```python
from build123d import *

# Parameters (mm, degrees)
SKETCH1_R               = 2.75
SKETCH1_R_2             = 1.5
BOSS_EXTRUDE1_DEPTH     = 4.5
SKETCH2_R               = 2.75
BOSS_EXTRUDE2_DEPTH     = 1
SKETCH4_R               = 3.75
BOSS_EXTRUDE3_DEPTH     = 6
CUT_EXTRUDE2_DEPTH      = 14.578475761
CUT_EXTRUDE2_DEPTH_BACK = 14.578475761
CUT_EXTRUDE3_DEPTH      = 14.336978811
CUT_EXTRUDE3_DEPTH_BACK = 14.336978811
CUT_EXTRUDE4_DEPTH      = 14.336978811
CUT_EXTRUDE4_DEPTH_BACK = 14.336978811
SKETCH7_R               = 1.5
SKETCH9_R               = 1.5
CUT_EXTRUDE5_DEPTH      = 14.336978811


with BuildPart() as part:
    # Sketch1 → Boss-Extrude1 (new body)
    with BuildSketch(Plane(origin=(0, 0, 0), x_dir=(1, 0, 0), z_dir=(0, 1, 0))):
        with Locations(Location((0, 0, 0), (0, 0, 270))):
            Circle(SKETCH1_R)
        with Locations(Location((0, 0, 0), (0, 0, 270))):
            Circle(SKETCH1_R_2, mode=Mode.SUBTRACT)
    extrude(amount=BOSS_EXTRUDE1_DEPTH)

    # Sketch2 → Boss-Extrude2 (add)
    with BuildSketch(Plane(origin=(0, 4.5, 0), x_dir=(1, 0, 0), z_dir=(0, 1, 0))):
        with Locations(Location((0, 0, 0), (0, 0, 270))):
            Circle(SKETCH2_R)
    extrude(amount=BOSS_EXTRUDE2_DEPTH)

    # Loft1: read off the stored shape, not the designer's step
    # Loft1: loft between two sections, ruled curve by curve
    loft1_from = [
        Edge.make_bspline([(-2.7249459, 5.5, -0.370364471), (-3.465674842, 5.5, 5.079527329), (1.984216958, 5.5, 5.820256271), (2.7249459, 5.5, 0.370364471), (3.465674842, 5.5, -5.079527329), (-1.984216958, 5.5, -5.820256271), (-2.7249459, 5.5, -0.370364471)], [0, 0, 0, 0, 0.5, 0.5, 0.5, 1, 1, 1, 1], 3, [1, 0.333333333, 0.333333333, 1, 0.333333333, 0.333333333, 1]),
    ]
    loft1_to = [
        Edge.make_bspline([(-3.66375351, 6.5, 0.799631301), (-2.064490908, 6.5, 8.127138321), (5.263016112, 6.5, 6.527875719), (3.66375351, 6.5, -0.799631301), (2.064490908, 6.5, -8.127138321), (-5.263016112, 6.5, -6.527875719), (-3.66375351, 6.5, 0.799631301)], [0, 0, 0, 0, 0.5, 0.5, 0.5, 1, 1, 1, 1], 3, [1, 0.333333333, 0.333333333, 1, 0.333333333, 0.333333333, 1]),
    ]
    loft1 = Solid(Shell([*[Face.make_surface_from_curves(loft1_from[k], loft1_to[k]) for k in range(1)], Face(Wire(loft1_from)), Face(Wire(loft1_to))]))
    add(loft1)

    # Sketch4 → Boss-Extrude3 (add)
    with BuildSketch(Plane(origin=(0, 6.5, 0), x_dir=(1, 0, 0), z_dir=(0, 1, 0))):
        with Locations(Location((0, 0, 0), (0, 0, 192.312))):
            Circle(SKETCH4_R)
    extrude(amount=BOSS_EXTRUDE3_DEPTH)

    # Sketch5 → Cut-Extrude2 (cut, two sides: drawn at the far end of the back side and taken through both)
    with BuildSketch(Plane(origin=(0, 0, 0), x_dir=(0, 0, -1), z_dir=(1, 0, 0)).offset(-CUT_EXTRUDE2_DEPTH_BACK)):
        with BuildLine():
            Line((2.35, 10.15), (2.35, 6.5))
            ThreePointArc((2.35, 6.5), (2.453708798, 5.961483519), (2.75, 5.5))
            Line((2.75, 5.5), (3.75, 6.5))
            Line((3.75, 6.5), (3.75, 12.5))
            Line((3.75, 12.5), (0, 12.5))
            ThreePointArc((0, 12.5), (1.661700936, 11.811700936), (2.35, 10.15))
        make_face()
        with BuildLine():
            ThreePointArc((-2.35, 10.15), (-1.661700936, 11.811700936), (0, 12.5))
            Line((0, 12.5), (-3.75, 12.5))
            Line((-3.75, 12.5), (-3.75, 6.5))
            Line((-3.75, 6.5), (-2.75, 5.5))
            ThreePointArc((-2.75, 5.5), (-2.453708798, 5.961483519), (-2.35, 6.5))
            Line((-2.35, 6.5), (-2.35, 10.15))
        make_face()
    extrude(amount=CUT_EXTRUDE2_DEPTH + CUT_EXTRUDE2_DEPTH_BACK, mode=Mode.SUBTRACT)

    # Sketch6 → Cut-Extrude3 (cut, two sides: drawn at the far end of the back side and taken through both)
    with BuildSketch(Plane.XY.offset(-CUT_EXTRUDE3_DEPTH_BACK)):
        with BuildLine():
            Line((2.75, 8.25), (2.75, 12.5))
            Line((2.75, 12.5), (-2.75, 12.5))
            Line((-2.75, 12.5), (-2.75, 8.25))
            ThreePointArc((-2.75, 8.25), (0, 5.5), (2.75, 8.25))
        make_face()
    extrude(amount=CUT_EXTRUDE3_DEPTH + CUT_EXTRUDE3_DEPTH_BACK, mode=Mode.SUBTRACT)

    # Sketch7 → Cut-Extrude4 (cut, two sides: drawn at the far end of the back side and taken through both)
    with BuildSketch(Plane(origin=(0, 0, 0), x_dir=(0, 0, -1), z_dir=(1, 0, 0)).offset(-CUT_EXTRUDE4_DEPTH_BACK)):
        with Locations((0, 10.3)):
            Circle(SKETCH7_R)
    extrude(amount=CUT_EXTRUDE4_DEPTH + CUT_EXTRUDE4_DEPTH_BACK, mode=Mode.SUBTRACT)

    # Sketch9 → Cut-Extrude5 (cut, through all)
    with BuildSketch(Plane.XY):
        with Locations(Location((0, 2.5, 0), (0, 0, 180))):
            Circle(SKETCH9_R)
    extrude(amount=CUT_EXTRUDE5_DEPTH, mode=Mode.SUBTRACT)


solid = part.part
```
Could you check a few things on this model? Use its own coordinates, in mm. A direction names the side the tool comes from. Give positions to 0.01 mm unless a question says otherwise; leave off trailing zeros. Loops run counter-clockwise (first coordinate to the right, second up) from the corner with the lowest first, then second, coordinate; pieces in that order, holes last. Notation, with made-up numbers: (-3.5, 12.5) - (15.5, 12.5) arc R25 cw to (15.5, 51.5) - close; hole circle Ø7 at (41.5, -20.75). An arc over 180 degrees is marked (long way). Answer in a Markdown table with one row per item. Add a question column.
Q1. We'd pull the mould along X, two halves only. Please class faces 1 (the face through (2.75, 10, 2)), 2 (the face through (0.121, 2.712, -2.747)), 3 (the face through (1.5, 2.43, 1.66)), 4 (the face through (-1.2, 0, 1.2)): +X half, -X half, draft (parallel to the pull), parting line (faces both ways), or undercut.
Q2. If we section it at C-C (y = 9): List the corners of the cut face in (x, z) for me.
Q3. If we section it at B-B (z = 0.3): State how many separate pieces and enclosed holes the cut face has, plus the area to 3 significant figures.
Q4. For pin 1 (2 mm diameter, centred on y = 1.5, z = -1, fed in from -X); pin 2 (0.6 mm diameter, centred on x = 2.5, y = 8, fed in from -Z); pin 3 (0.9 mm diameter, centred on x = -2.5, y = 8, fed in from +Z), each with a flat end and sliding along its axis, tell me the tip position at first contact or that it passes through.
Q5. Please list where these lines run through material, in increasing order: L1, parallel to X at y = 2.5, z = 1.75; L2, parallel to Y at x = 0, z = 1.6; L3, parallel to X at y = 2.4, z = 0. Write a range as from..to.
Q6. If we section it at A-A (y = 10.3): List the corners of the cut face in (x, z) for me, plus the area to 3 significant figures.
Q7. Which directions (+Z, -Z, +X, -X, +Y, -Y) give clear straight access to the entire face, cutting with the end or side of a thin tool? Please do faces 5 (the face through (-2.75, 9, -1.1)), 6 (the face through (-3.75, 8.12, -0.04)).
Q8. If we section it at D-D (y = 2): List the corners of the cut face in (x, z) for me.
The answers:
| question | item | result |
|---|---|---|
| 1 | face 1 | undercut |
| 1 | face 2 | parting line |
| 1 | face 3 | undercut |
| 1 | face 4 | draft |
| 2 | outline | (-3.67, -0.75) arc R3.75 ccw to (-2.92, -2.35) - (-2.75, -2.35) - (-2.75, -0.75) - close; (-3.67, 0.75) - (-2.75, 0.75) - (-2.75, 2.35) - (-2.92, 2.35) arc R3.75 ccw to start; (2.75, -2.35) - (2.92, -2.35) arc R3.75 ccw to (3.67, -0.75) - (2.75, -0.75) - close; (2.75, 0.75) - (3.67, 0.75) arc R3.75 ccw to (2.92, 2.35) - (2.75, 2.35) - close |
| 3 | separate pieces | 3 |
| 3 | enclosed holes | 0 |
| 3 | area | 27.0 mm^2 |
| 4 | pin 1 | stops at x = -2.75 |
| 4 | pin 2 | stops at z = -2.35 |
| 4 | pin 3 | stops at z = 2.35 |
| 5 | L1 | x = -2.12..-1.5, 1.5..2.12 |
| 5 | L2 | y = 0..1, 4..5.5 |
| 5 | L3 | x = -2.75..-1.5, 1.5..2.75 |
| 6 | outline | (-3.44, -1.5) arc R3.75 ccw to (-2.93, -2.35) - (-2.75, -2.35) - (-2.75, -1.5) - close; (-3.44, 1.5) - (-2.75, 1.5) - (-2.75, 2.35) - (-2.93, 2.35) arc R3.75 ccw to start; (2.75, -2.35) - (2.93, -2.35) arc R3.75 ccw to (3.44, -1.5) - (2.75, -1.5) - close; (2.75, 1.5) - (3.44, 1.5) arc R3.75 ccw to (2.93, 2.35) - (2.75, 2.35) - close |
| 6 | area | 1.55 mm^2 |
| 7 | face 5 | +Z, -Z, +Y |
| 7 | face 6 | -X, +Y, -Y |
| 8 | outline | (-1.41, 0.5) - (-1.41, 2.36) arc R2.75 ccw (long way) to (1.41, 2.36) - (1.41, 0.5) arc R1.5 cw (long way) to start |
